```python
from build123d import *

# Parameters (mm, degrees)
F1_DEPTH      = 2
F3_DEPTH      = 2.2
F5_DEPTH      = 25
F6_R          = 1.5
F7_DEPTH      = 4.2
F8_R          = 2.75
F9_DEPTH      = 1.6
F10_S5_R      = 1.5
F10_T6_DEPTH  = 5
F10_S11_R     = 1.5
F10_T12_DEPTH = 5
F10_S17_R     = 1.5
F10_T18_DEPTH = 5
F10_S23_R     = 1.5
F10_T24_DEPTH = 5
F11_W         = 5.6
F11_H         = 2
F12_DEPTH     = 0.4
F13_T1_DEPTH  = 8.0494897428
F13_T3_DEPTH  = 8.0494897428


# Not quite as in the source:
# - a fillet or chamfer that OpenCascade refuses, or shapes differently, is made with other operations: its cross-section is extruded or revolved along the edge and cut away or added


with BuildPart() as f1:
    # F0 (on Top) → F1 (new body)
    with BuildSketch(Plane.XY):
        with BuildLine():
            Line((80, 0), (2, 0))
            ThreePointArc((2, 0), (0.5857864376, -0.5857864376), (0, -2))
            Line((0, -2), (0, -88))
            ThreePointArc((0, -88), (0.5857864376, -89.4142135624), (2, -90))
            Line((2, -90), (11.25, -90))
            Line((11.25, -90), (11.25, -62.5))
            Line((11.25, -62.5), (15.8564011104, -56.3307127986))
            ThreePointArc((15.8564011104, -56.3307127986), (16.5951030311, -54.9153368199), (16.85, -53.3392666362))
            Line((16.85, -53.3392666362), (16.85, -26))
            ThreePointArc((16.85, -26), (17.4357864376, -24.5857864376), (18.85, -24))
            Line((18.85, -24), (63.15, -24))
            ThreePointArc((63.15, -24), (64.5642135624, -24.5857864376), (65.15, -26))
            Line((65.15, -26), (65.15, -53.3392666362))
            ThreePointArc((65.15, -53.3392666362), (65.4048969689, -54.9153368199), (66.1435988896, -56.3307127986))
            Line((66.1435988896, -56.3307127986), (70.75, -62.5))
            Line((70.75, -62.5), (70.75, -90))
            Line((70.75, -90), (80, -90))
            ThreePointArc((80, -90), (81.4142135624, -89.4142135624), (82, -88))
            Line((82, -88), (82, -2))
            ThreePointArc((82, -2), (81.4142135624, -0.5857864376), (80, 0))
        make_face()
    extrude(amount=F1_DEPTH)

    # F2 (on face) → F3 (join)
    with BuildSketch(Plane(origin=(0, 0, 0), x_dir=(1, 0, 0), z_dir=(0, 0, -1))):
        with BuildLine():
            ThreePointArc((80, 0), (81.4142135624, 0.5857864376), (82, 2))
            Line((82, 2), (82, 88))
            ThreePointArc((82, 88), (81.4142135624, 89.4142135624), (80, 90))
            Line((80, 90), (70.75, 90))
            Line((70.75, 90), (70.75, 62.5))
            Line((70.75, 62.5), (70.75, 26))
            ThreePointArc((70.75, 26), (70.1642135624, 24.5857864376), (68.75, 24))
            Line((68.75, 24), (65.15, 24))
            Line((65.15, 24), (16.85, 24))
            Line((16.85, 24), (13.25, 24))
            ThreePointArc((13.25, 24), (11.8357864376, 24.5857864376), (11.25, 26))
            Line((11.25, 26), (11.25, 62.5))
            Line((11.25, 62.5), (11.25, 90))
            Line((11.25, 90), (2, 90))
            ThreePointArc((2, 90), (0.5857864376, 89.4142135624), (0, 88))
            Line((0, 88), (0, 2))
            ThreePointArc((0, 2), (0.5857864376, 0.5857864376), (2, 0))
            Line((2, 0), (80, 0))
        make_face()
    extrude(amount=F3_DEPTH)

    # F4 (on face) → F5 (cut)
    with BuildSketch(Plane.XY.offset(2)):
        with BuildLine():
            Line((18.3, -2), (10.5, -2))
            Line((10.5, -2), (10.5, -7.6))
            ThreePointArc((10.5, -7.6), (11.0857864376, -9.0142135624), (12.5, -9.6))
            Line((12.5, -9.6), (16.3, -9.6))
            ThreePointArc((16.3, -9.6), (17.7142135624, -9.0142135624), (18.3, -7.6))
            Line((18.3, -7.6), (18.3, -2))
        make_face()
    extrude(amount=-F5_DEPTH, mode=Mode.SUBTRACT)

    # F6 (on face) → F7 (cut)
    with BuildSketch(Plane.XY.offset(2)):
        with Locations((5.5, -84.5)):
            Circle(F6_R)
        with Locations((76.5, -84.5)):
            Circle(F6_R)
        with Locations((5.5, -5.5)):
            Circle(F6_R)
        with Locations((76.5, -5.5)):
            Circle(F6_R)
    extrude(amount=-F7_DEPTH, mode=Mode.SUBTRACT)

    # F8 (on face) → F9 (cut)
    with BuildSketch(Plane.XY.offset(2)):
        with Locations((5.5, -5.5)):
            Circle(F8_R)
        with Locations((76.5, -5.5)):
            Circle(F8_R)
        with Locations((76.5, -84.5)):
            Circle(F8_R)
        with Locations((5.5, -84.5)):
            Circle(F8_R)
    extrude(amount=-F9_DEPTH, mode=Mode.SUBTRACT)

    # F10: chamfer of 1.5 on 4 edges, made by hand


with BuildPart() as f10_tool2:
    # F10_s3 → F10_t4 (revolve)
    with BuildSketch(Plane.XZ.offset(84.5)):
        Polygon((8.25, 1.9), (6.75, 0.4), (8.25, 0.4), align=None)
    revolve(axis=Axis((5.5, -84.5, 0.4), (0, 0, 1)))

    # F10_s5 → F10_t6 (cut, symmetric)
    with BuildSketch(Plane.XY.offset(1.1)):
        with Locations((5.5, -84.5)):
            Circle(F10_S5_R)
    extrude(amount=F10_T6_DEPTH, both=True, mode=Mode.SUBTRACT)


with BuildPart() as f1_1:
    add(f1.part)

    # F10_t1: union F10_tool2
    add(f10_tool2.part)


with BuildPart() as f10_tool8:
    # F10_s9 → F10_t10 (revolve)
    with BuildSketch(Plane.XZ.offset(84.5)):
        Polygon((79.25, 1.9), (77.75, 0.4), (79.25, 0.4), align=None)
    revolve(axis=Axis((76.5, -84.5, 0.4), (0, 0, 1)))

    # F10_s11 → F10_t12 (cut, symmetric)
    with BuildSketch(Plane.XY.offset(1.1)):
        with Locations((76.5, -84.5)):
            Circle(F10_S11_R)
    extrude(amount=F10_T12_DEPTH, both=True, mode=Mode.SUBTRACT)


with BuildPart() as f1_2:
    add(f1_1.part)

    # F10_t7: union F10_tool8
    add(f10_tool8.part)


with BuildPart() as f10_tool14:
    # F10_s15 → F10_t16 (revolve)
    with BuildSketch(Plane.XZ.offset(5.5)):
        Polygon((8.25, 1.9), (6.75, 0.4), (8.25, 0.4), align=None)
    revolve(axis=Axis((5.5, -5.5, 0.4), (0, 0, 1)))

    # F10_s17 → F10_t18 (cut, symmetric)
    with BuildSketch(Plane.XY.offset(1.1)):
        with Locations((5.5, -5.5)):
            Circle(F10_S17_R)
    extrude(amount=F10_T18_DEPTH, both=True, mode=Mode.SUBTRACT)


with BuildPart() as f1_3:
    add(f1_2.part)

    # F10_t13: union F10_tool14
    add(f10_tool14.part)


with BuildPart() as f10_tool20:
    # F10_s21 → F10_t22 (revolve)
    with BuildSketch(Plane.XZ.offset(5.5)):
        Polygon((79.25, 1.9), (77.75, 0.4), (79.25, 0.4), align=None)
    revolve(axis=Axis((76.5, -5.5, 0.4), (0, 0, 1)))

    # F10_s23 → F10_t24 (cut, symmetric)
    with BuildSketch(Plane.XY.offset(1.1)):
        with Locations((76.5, -5.5)):
            Circle(F10_S23_R)
    extrude(amount=F10_T24_DEPTH, both=True, mode=Mode.SUBTRACT)


with BuildPart() as f1_4:
    add(f1_3.part)

    # F10_t19: union F10_tool20
    add(f10_tool20.part)

    # F11 (on face) → F12 (join)
    with BuildSketch(Plane(origin=(0, 0, 0), x_dir=(1, 0, 0), z_dir=(0, 0, -1))):
        with Locations((14.05, 43.5)):
            Rectangle(F11_W, F11_H)
        with Locations((67.95, 43.5)):
            Rectangle(F11_W, F11_H)
    extrude(amount=F12_DEPTH)

    # F13: fillet of radius 1.4 on 4 edges, made by hand

    # F13_s2 → F13_t1 (cut)
    with BuildSketch(Plane.YZ.offset(11.25)):
        with BuildLine():
            ThreePointArc((-42.5, 0), (-42.9506456349, -0.2961481397), (-43.4797958971, -0.4))
            Line((-43.4797958971, -0.4), (-42.5, -0.4))
            Line((-42.5, -0.4), (-42.5, 0))
        make_face()
        with BuildLine():
            ThreePointArc((-43.5202041029, -0.4), (-44.0493543651, -0.2961481397), (-44.5, 0))
            Line((-44.5, 0), (-44.5, -0.4))
            Line((-44.5, -0.4), (-43.5202041029, -0.4))
        make_face()
    extrude(amount=F13_T1_DEPTH, mode=Mode.SUBTRACT)

    # F13_s4 → F13_t3 (cut)
    with BuildSketch(Plane.YZ.offset(62.7005102572)):
        with BuildLine():
            ThreePointArc((-43.4797958971, -0.4), (-42.9506456349, -0.2961481397), (-42.5, 0))
            Line((-42.5, 0), (-42.5, -0.4))
            Line((-42.5, -0.4), (-43.4797958971, -0.4))
        make_face()
        with BuildLine():
            ThreePointArc((-44.5, 0), (-44.0493543651, -0.2961481397), (-43.5202041029, -0.4))
            Line((-43.5202041029, -0.4), (-44.5, -0.4))
            Line((-44.5, -0.4), (-44.5, 0))
        make_face()
    extrude(amount=F13_T3_DEPTH, mode=Mode.SUBTRACT)


solid = f1_4.part
```
The listing builds one solid part. Answer for the finished solid, in the listing's coordinates (mm). A direction names the side the tool comes from. Coordinates: 2 decimals unless noted, no trailing zeros. Loops run counter-clockwise (first coordinate to the right, second up) from the corner with the lowest first, then second, coordinate; pieces in that order, holes last. Notation, with made-up numbers: (14, -23.5) - (72, -23.5) arc R27 ccw to (72, 6.5) - close; hole circle Ø9 at (48.25, 84). An arc over 180 degrees is marked (long way). Use a Markdown table: item, result. Add a question column.
1) The part is cut by section C-C, the plane y = -33. Give the vertices of the cut face in (x, z).
2) The part is cut by section B-B, the plane x = 76.5. Give the vertices of the cut face in (y, z), and give its area (3 significant figures).
3) The part is cut by section A-A, the plane y = -84.5. Give the vertices of the cut face in (x, z).
4) The part is cut by section D-D, the plane z = -1.35. Give the vertices of the cut face in (x, y), and give its area (3 significant figures).
5) Given pin 1 (5 mm diameter, centred on x = 76.5, y = -84.5, fed in from +Z); pin 2 (3.5 mm diameter, centred on x = 5.5, y = -84.5, fed in from +Z); pin 3 (7 mm diameter, centred on x = 76.5, y = -5.5, fed in from -Z); pin 4 (1.3 mm diameter, centred on x = 36.5, z = -0.5, fed in from -Y), each flat-ended and moving along its own axis, determine where each tip first touches the part or whether it passes through.
6) Find the intervals of material crossed by line 1 (Y direction, x = 76.5, z = -0.9); line 2 (X direction, y = -84.5, z = -0.95); line 3 (X direction, y = -45, z = -1.55), in increasing order.
7) For faces 1 (the flat face through (14, -2, 0)), 2 (the cylindrical face through (70.18, -24.6, -1.08)), 3 (the flat face through (16.85, -40, 1)), 4 (the cylindrical face through (0.57, -0.6, -0.07)), 5 (the flat face through (0, -46, 0)), determine the directions among +Z, -Z, +X, -X, +Y, -Y from which every point of the face is accessible in a straight line to the end or side of a thin tool.
8) The mould has two halves that part along Y. Classify faces 6 (the flat face through (14, -51, 0)), 7 (the flat face through (68, -33, 0)), 8 (the flat face through (68.415, -59.372, 0.986)): released by +Y, released by -Y, zero draft, split by the parting line, or undercut.
Here are the results:
| question | item | result |
|---|---|---|
| 1 | outline | (0, -2.2) - (11.25, -2.2) - (11.25, 0) - (16.85, 0) - (16.85, 2) - (0, 2) - close; (65.15, 0) - (70.75, 0) - (70.75, -2.2) - (82, -2.2) - (82, 2) - (65.15, 2) - close |
| 2 | outline | (-90, -2.2) - (-86, -2.2) - (-86, 0.65) - (-87.25, 1.9) - (-87.25, 2) - (-90, 2) - close; (-83, -2.2) - (-7, -2.2) - (-7, 0.65) - (-8.25, 1.9) - (-8.25, 2) - (-81.75, 2) - (-81.75, 1.9) - (-83, 0.65) - close; (-4, -2.2) - (0, -2.2) - (0, 2) - (-2.75, 2) - (-2.75, 1.9) - (-4, 0.65) - close |
| 2 | area | 349 mm^2 |
| 3 | outline | (0, -2.2) - (4, -2.2) - (4, 0.65) - (2.75, 1.9) - (2.75, 2) - (0, 2) - close; (7, -2.2) - (11.25, -2.2) - (11.25, 2) - (8.25, 2) - (8.25, 1.9) - (7, 0.65) - close; (70.75, -2.2) - (75, -2.2) - (75, 0.65) - (73.75, 1.9) - (73.75, 2) - (70.75, 2) - close; (78, -2.2) - (82, -2.2) - (82, 2) - (79.25, 2) - (79.25, 1.9) - (78, 0.65) - close |
| 4 | outline | (0, -88) arc R2 ccw to (2, -90) - (11.25, -90) - (11.25, -26) arc R2 cw to (13.25, -24) - (68.75, -24) arc R2 cw to (70.75, -26) - (70.75, -90) - (80, -90) arc R2 ccw to (82, -88) - (82, -2) arc R2 ccw to (80, 0) - (2, 0) arc R2 ccw to (0, -2) - close; hole circle Ø3 at (5.5, -84.5); hole circle Ø3 at (5.5, -5.5); hole (10.5, -7.6) arc R2 ccw to (12.5, -9.6) - (16.3, -9.6) arc R2 ccw to (18.3, -7.6) - (18.3, -2) - (10.5, -2) - close; hole circle Ø3 at (76.5, -84.5); hole circle Ø3 at (76.5, -5.5) |
| 4 | area | 3,370 mm^2 |
| 5 | pin 1 | stops at z = 1.65 |
| 5 | pin 2 | stops at z = 0.9 |
| 5 | pin 3 | stops at z = -2.2 |
| 5 | pin 4 | stops at y = -24 |
| 6 | line 1 | y = -90 to -86, -83 to -7, -4 to 0 |
| 6 | line 2 | x = 0 to 4, 7 to 11.25, 70.75 to 75, 78 to 82 |
| 6 | line 3 | x = 0 to 11.25, 70.75 to 82 |
| 7 | face 1 | +Z, -Z |
| 7 | face 2 | -Z |
| 7 | face 3 | +Z, -Z, -Y |
| 7 | face 4 | +Z, -Z, -X, +Y |
| 7 | face 5 | +Z, -Z, -X, +Y, -Y |
| 8 | face 6 | zero draft |
| 8 | face 7 | undercut |
| 8 | face 8 | released by -Y |
